Build history of the part. All positions in model axes, mm. Round coordinates to 2 decimals unless told otherwise and drop trailing zeros. Write each loop counter-clockwise with the first axis right and the second up, starting at its lowest first coordinate (ties: lowest second). Pieces come first, ordered by that corner, then holes.
from build123d import *
from OCP.BRepFilletAPI import BRepFilletAPI_MakeChamfer

# Parameters (mm, degrees)
SKETCH1_W                  = 300
SKETCH1_H                  = 300
BOSS_EXTRUDE1_DEPTH        = 300
SKETCH3_R                  = 110
BOSS_EXTRUDE2_DEPTH        = 10
SKETCH4_R                  = 5
BOSS_EXTRUDE3_DEPTH        = 10
CHAMFER1_SIZE              = 2
CHAMFER2_SIZE              = 2
M10X1_0_TAPPED_HOLE1_D     = 9
M10X1_0_TAPPED_HOLE1_DEPTH = 23
M10X1_0_TAPPED_HOLE1_TIP   = 2.703872786
SKETCH7_W                  = 20
SKETCH7_H                  = 40
BOSS_EXTRUDE4_DEPTH        = 300
CHAMFER3_SIZE              = 3
CHAMFER3_SIZE2             = 3.575260778
M6_CLEARANCE_HOLE1_D       = 6.6


with BuildPart() as part:
    # Sketch1 → Boss-Extrude1 (new body)
    with BuildSketch(Plane(origin=(0, 0, 0), x_dir=(1, 0, 0), z_dir=(0, 1, 0))):
        Rectangle(SKETCH1_W, SKETCH1_H)
    extrude(amount=BOSS_EXTRUDE1_DEPTH)

    # Sketch2 → Cut-Revolve1 (revolve, cut)
    with BuildSketch(Plane.XY, mode=Mode.PRIVATE) as cut_revolve1_sk:
        Polygon((110, 300), (250, 219.170962313), (250, 300), align=None)
    revolve(cut_revolve1_sk.sketch.rotate(Axis((0, 394.192122867, 0), (0, -1, 0)), 314.999999708), axis=Axis((0, 394.192122867, 0), (0, -1, 0)), mode=Mode.SUBTRACT)

    # Sketch3 → Boss-Extrude2 (add)
    with BuildSketch(Plane(origin=(0, 300, 0), x_dir=(1, 0, 0), z_dir=(0, 1, 0))):
        with Locations(Location((0, 0, 0), (0, 0, 270))):
            Circle(SKETCH3_R)
    extrude(amount=BOSS_EXTRUDE2_DEPTH)

    # Sketch4 → Boss-Extrude3 (add)
    with BuildSketch(Plane(origin=(0, 310, 0), x_dir=(1, 0, 0), z_dir=(0, 1, 0))):
        with Locations(Location((80, 0, 0), (0, 0, 270))):
            Circle(SKETCH4_R)
    extrude(amount=BOSS_EXTRUDE3_DEPTH)

    # Chamfer1
    chamfer1_edges = [part.edges().sort_by_distance(p)[0] for p in [
        (0, 310, -110),
    ]]
    chamfer(chamfer1_edges, length=CHAMFER1_SIZE)

    # Chamfer2
    chamfer2_edges = [part.edges().sort_by_distance(p)[0] for p in [
        (80, 320, -5),
    ]]
    chamfer(chamfer2_edges, length=CHAMFER2_SIZE)

    # M10x1.0 Tapped Hole1
    with Locations(Plane(origin=(0, 310, 0), x_dir=(1, 0, 0), z_dir=(0, 1, 0))):
        with Locations((0, 0)):
            Hole(M10X1_0_TAPPED_HOLE1_D / 2, depth=M10X1_0_TAPPED_HOLE1_DEPTH)
            with Locations((0, 0, -(M10X1_0_TAPPED_HOLE1_DEPTH + M10X1_0_TAPPED_HOLE1_TIP / 2))):  # 118° drill point
                Cone(0, M10X1_0_TAPPED_HOLE1_D / 2, M10X1_0_TAPPED_HOLE1_TIP, mode=Mode.SUBTRACT)

    # Sketch7 → Boss-Extrude4 (add)
    with BuildSketch(Plane.XY.offset(150)):
        with Locations((-10, 180)):
            Rectangle(SKETCH7_W, SKETCH7_H)
    extrude(amount=BOSS_EXTRUDE4_DEPTH)

    # Chamfer3: one chamfer whose edges measure the first distance from different faces: ONE call of the kernel's chamfer builder (chamfer() names one face for all edges)
    chamfer3_edges_1 = [part.edges().sort_by_distance(p)[0] for p in [
        (-10, 200, 450),
    ]]
    chamfer3_side_1 = [part.faces().sort_by_distance(p)[0] for p in [
        (-10, 200, 300),
    ]]
    chamfer3_edges_2 = [part.edges().sort_by_distance(p)[0] for p in [
        (-10, 160, 450),
    ]]
    chamfer3_side_2 = [part.faces().sort_by_distance(p)[0] for p in [
        (-10, 160, 300),
    ]]
    chamfer3 = BRepFilletAPI_MakeChamfer(part.part.solid().wrapped)
    for e in chamfer3_edges_1:
        chamfer3.Add(CHAMFER3_SIZE, CHAMFER3_SIZE2, e.wrapped, chamfer3_side_1[0].wrapped)  # the first distance lies on this face
    for e in chamfer3_edges_2:
        chamfer3.Add(CHAMFER3_SIZE, CHAMFER3_SIZE2, e.wrapped, chamfer3_side_2[0].wrapped)  # the first distance lies on this face
    add(Compound.cast(chamfer3.Shape()), mode=Mode.REPLACE)

    # M6 Clearance Hole1 (through all)
    with Locations(Plane(origin=(0, 0, 0), x_dir=(0, 0, -1), z_dir=(1, 0, 0))):
        with Locations((-444, 180), (-294, 180)):
            Hole(M6_CLEARANCE_HOLE1_D / 2)


solid = part.part
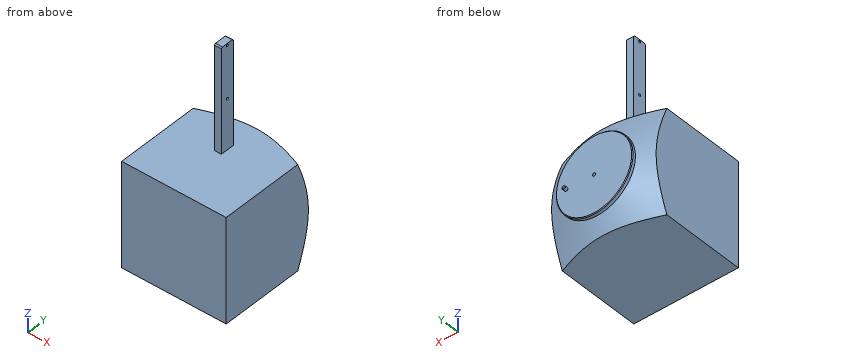
1) Wall check: L1, parallel to Z at x = -6, y = 180; L2, parallel to Z at x = 0, y = 303; L3, parallel to Y at x = -5, z = 294. Give the ranges that are in metal, low to high.
Results:
L1: z = -150 to 290.7, 297.3 to 440.7, 447.3 to 450
L2: z = -110 to -4.5, 4.5 to 110
L3: y = 160 to 176.7, 183.3 to 200
2) Slice it at A-A (y = 224). Write the cut outline in (x, z), plus the area to 3 significant figures.
Results:
outline: (-150, -150) - (150, -150) - (150, 150) - (-150, 150) - close
area: 90,000 mm2
3) Pin check, flat tips, straight feed: pin 1 Ø8.5 at (y, z) = (180, 444) entering from +X; pin 2 Ø22 at (x, z) = (-15, 227) entering from +Y; pin 3 Ø8 at (x, y) = (117, 75.5) entering from +Z. Stop position of each tip, or through.
Results:
pin 1: stops at x = 0
pin 2: stops at y = 200
pin 3: stops at z = 150
